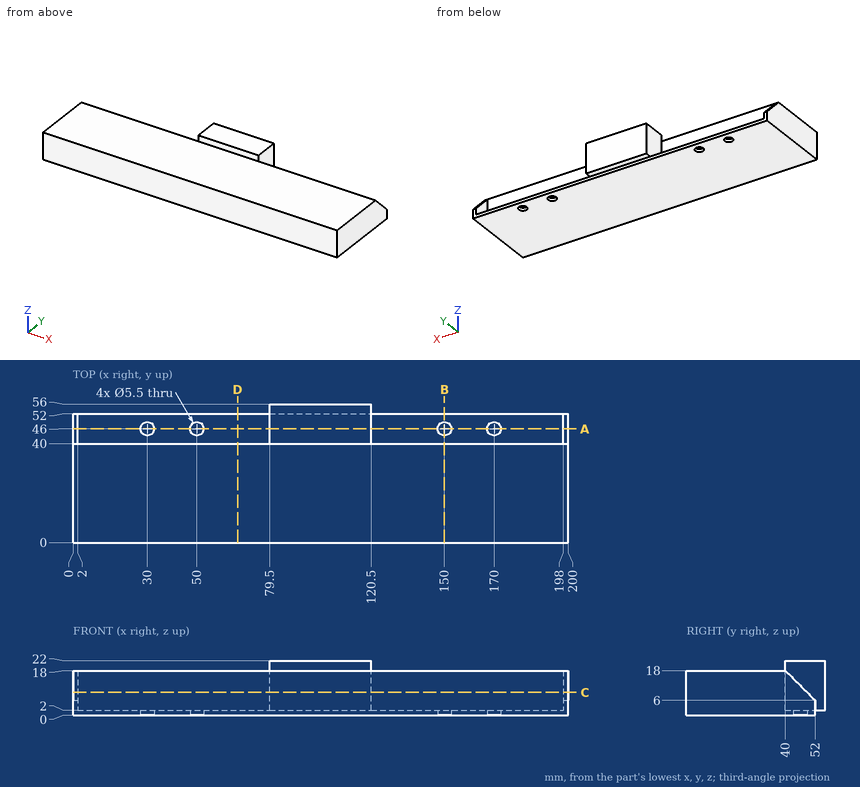
Here's the drawing with two shaded views (mm, measured from the low corner). I have some questions. Coordinates: 2 decimals unless noted, no trailing zeros. Write each loop counter-clockwise with the first axis right and the second up, starting at its lowest first coordinate (ties: lowest second). Pieces come first, ordered by that corner, then holes.
Item 1: I want a section at C-C on z = 9.25. Write out the boundary of the cut face in (x, y).
Item 2: If I drill on line 1 (X direction, y = 47, z = 6); line 2 (Y direction, x = 50, z = 1.5); line 3 (Y direction, x = 74.5, z = 1.5), over which ranges is the centre line in solid material (lowest first)?
Item 3: Will these pins go through, and if not, where does the flat tip stop? pin 1 (13 mm diameter, centred on x = 148, z = 12, fed in from +Y); pin 2 (3.5 mm diameter, centred on x = 29, y = 44, fed in from +Z); pin 3 (5 mm diameter, centred on x = 68.5, z = 4, fed in from +Y).
Item 4: I want a section at B-B on x = 150. Write out the boundary of the cut face in (y, z).
Item 5: I want a section at A-A on y = 46. Write out the boundary of the cut face in (x, z), and give its area (3 significant figures).
Item 6: I want a section at D-D on x = 66.5. Write out the boundary of the cut face in (y, z), and give its area (3 significant figures).
Findings below:
1. outline: (0, 0) - (200, 0) - (200, 48.75) - (198, 48.75) - (198, 40) - (120.5, 40) - (120.5, 56) - (79.5, 56) - (79.5, 40) - (2, 40) - (2, 48.75) - (0, 48.75) - close
2. line 1: x = 0 to 2, 79.5 to 120.5, 198 to 200
2. line 2: y = 0 to 43.25, 48.75 to 52
2. line 3: y = 0 to 52
3. pin 1: stops at y = 40
3. pin 2: stops at z = 2
3. pin 3: stops at y = 52
4. outline: (0, 0) - (43.25, 0) - (43.25, 2) - (40, 2) - (40, 18) - (0, 18) - close; (48.75, 0) - (52, 0) - (52, 2) - (48.75, 2) - close
5. outline: (0, 0) - (27.25, 0) - (27.25, 2) - (2, 2) - (2, 12) - (0, 12) - close; (32.75, 0) - (47.25, 0) - (47.25, 2) - (32.75, 2) - close; (52.75, 0) - (147.25, 0) - (147.25, 2) - (120.5, 2) - (120.5, 22) - (79.5, 22) - (79.5, 2) - (52.75, 2) - close; (152.75, 0) - (167.25, 0) - (167.25, 2) - (152.75, 2) - close; (172.75, 0) - (200, 0) - (200, 12) - (198, 12) - (198, 2) - (172.75, 2) - close
5. area: 1,220 mm2
6. outline: (0, 0) - (52, 0) - (52, 2) - (40, 2) - (40, 18) - (0, 18) - close
6. area: 744 mm2
